Source: three-view drawing plus pictorial views. Frame: mm from the lowest corner of the part. A direction names the side the tool comes from. Round coordinates to 2 decimals unless told otherwise and drop trailing zeros. Loops run counter-clockwise (first coordinate to the right, second up) from the corner with the lowest first, then second, coordinate; pieces in that order, holes last. Notation, with made-up numbers: M -11,-13 L 29,-13 A16 ccw 29,1 Z; hole C 21,-31 d2. An arc over 180 degrees is marked long. Return JSON: item names as keys, results as strings. Group by question number.
1) Section C-C (z = 26.5). Output: boundary loops of the cut face in (x, y), plus the area to 3 significant figures.
2) Access query for the marked faces 1 and 2. Directions: +Z, -Z, +X, -X, +Y, -Y. A direction counts if a zero-diameter tool reaches every point of the face in a straight line with its end or side. Return the directions, or none.
3) Section D-D (x = 5). Output: boundary loops of the cut face in (y, z), plus the area to 3 significant figures.
4) Section B-B (z = 8). Output: boundary loops of the cut face in (x, y), plus the area to 3 significant figures.
5) Material intervals for line 1 (X direction, y = 50, z = 8); line 2 (X direction, y = 25.5, z = 2.5); line 3 (Y direction, x = 11, z = 31.5), sorted ascending. Write a range as from..to.
6) Section A-A (x = 11). Output: boundary loops of the cut face in (y, z).
7) Contact query for flat-ended pins moving along their axis: P1, Ø1.5, axis at x = 6.5, z = 11.5, coming from the -Y side; P2, Ø24, axis at y = 29, z = 13.5, coming from the +X side. Output: stop coordinate, or through.
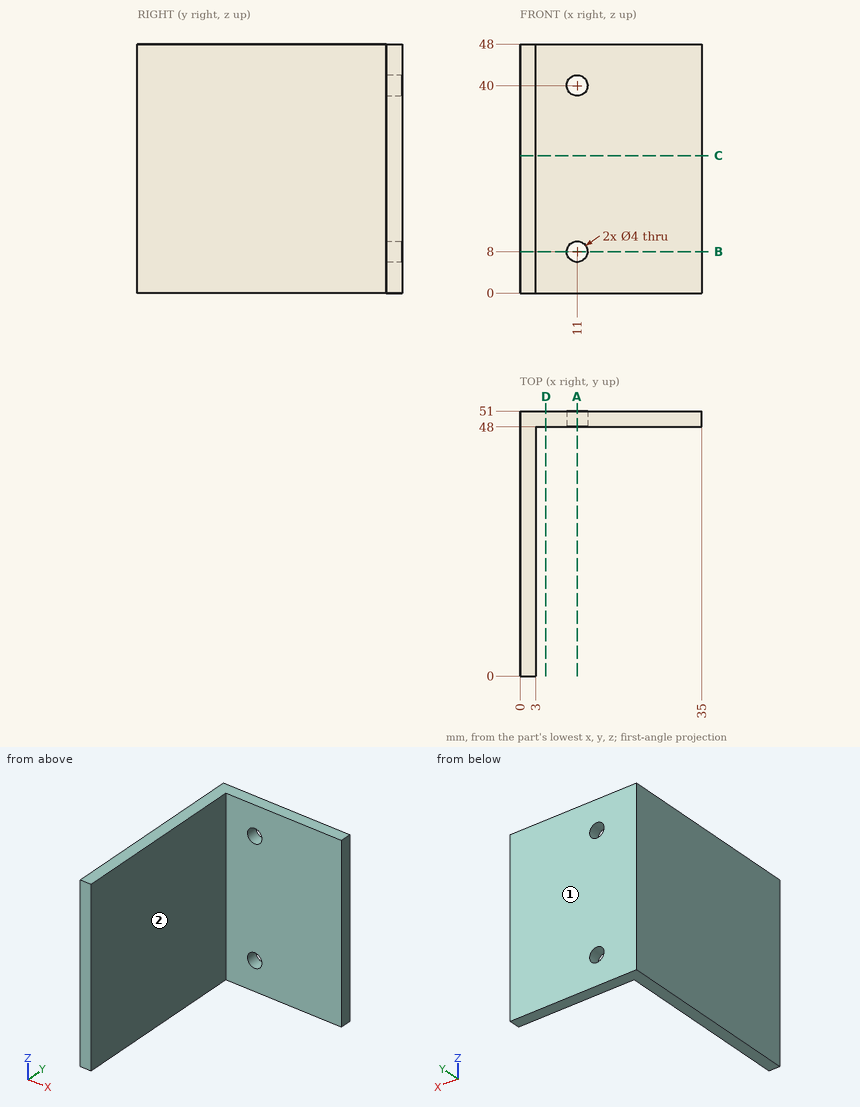
Returned:
{
 "1": {"outline": "M 0,0 L 3,0 L 3,48 L 35,48 L 35,51 L 0,51 Z", "area": "249 mm^2"},
 "2": {"face 1": "+Z, -Z, +X, -X, +Y", "face 2": "+Z, -Z, +X, -Y"},
 "3": {"outline": "M 48,0 L 51,0 L 51,48 L 48,48 Z", "area": "144 mm^2"},
 "4": {"outline": "M 0,0 L 3,0 L 3,48 L 9,48 L 9,51 L 0,51 Z; M 13,48 L 35,48 L 35,51 L 13,51 Z", "area": "237 mm^2"},
 "5": {"line 1": "x = 0..9, 13..35", "line 2": "x = 0..3", "line 3": "y = 48..51"},
 "6": {"outline": "M 48,0 L 51,0 L 51,6 L 48,6 Z; M 48,10 L 51,10 L 51,38 L 48,38 Z; M 48,42 L 51,42 L 51,48 L 48,48 Z"},
 "7": {"P1": "stops at y = 48", "P2": "stops at x = 3"}
}
